Job drawing, mm, ordinate dimensions from the low corner. One solid piece. Round coordinates to 2 decimals unless told otherwise and drop trailing zeros. Write each loop counter-clockwise with the first axis right and the second up, starting at its lowest first coordinate (ties: lowest second). Pieces come first, ordered by that corner, then holes.
1) Saw through at D-D (z = 43.5). Write the cut outline in (x, y).
2) Saw through at C-C (z = 23). Write the cut outline in (x, y), plus the area to 3 significant figures.
3) Saw through at A-A (x = 1.1). State how many separate pieces and enclosed holes the cut face has, plus the area to 3 significant figures.
4) Saw through at B-B (y = 37). Write the cut outline in (x, z).
5) Flat gauge pins, fed straight in: pin 1 (1.5 mm diameter, centred on x = 2.5, y = 30.5, fed in from +Z); pin 2 (2 mm diameter, centred on y = 35, z = 7, fed in from -X). Where does each tip first touch, or does it go through?
6) Wall check: probe 1 along Y at (x, z) = (1.95, 23); probe 2 along Z at (x, y) = (0.9, 23.5); probe 3 along Y at (x, z) = (2.2, 10). Give the ranges that are in metal, low to high.
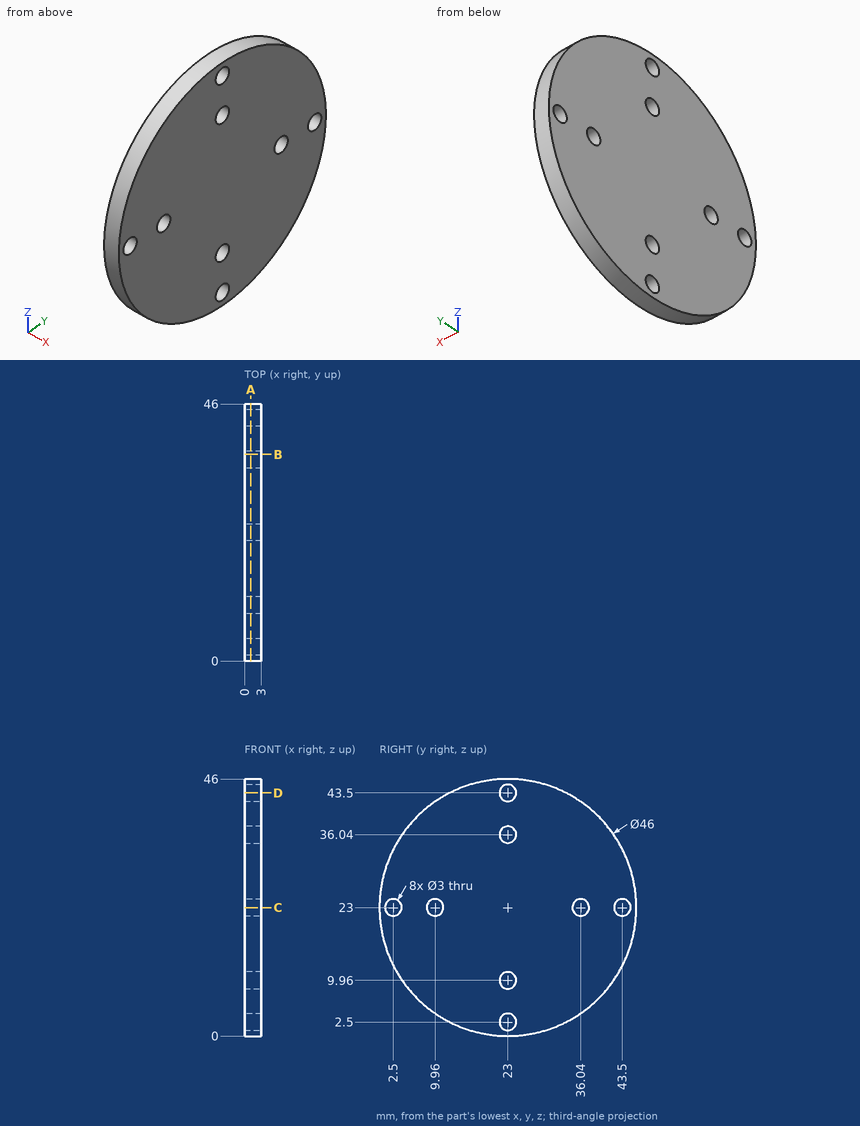
Evaluation:
1. outline: (0, 12.57) - (3, 12.57) - (3, 21.5) - (0, 21.5) - close; (0, 24.5) - (3, 24.5) - (3, 33.43) - (0, 33.43) - close
2. outline: (0, 0) - (3, 0) - (3, 1) - (0, 1) - close; (0, 4) - (3, 4) - (3, 8.46) - (0, 8.46) - close; (0, 11.46) - (3, 11.46) - (3, 34.54) - (0, 34.54) - close; (0, 37.54) - (3, 37.54) - (3, 42) - (0, 42) - close; (0, 45) - (3, 45) - (3, 46) - (0, 46) - close
2. area: 102 mm2
3. separate pieces: 1
3. enclosed holes: 8
3. area: 1,610 mm2
4. outline: (0, 4.75) - (3, 4.75) - (3, 21.85) - (0, 21.85) - close; (0, 24.15) - (3, 24.15) - (3, 41.25) - (0, 41.25) - close
5. pin 1: stops at z = 44.99
5. pin 2: stops at x = 0
6. probe 1: y = 0 to 1, 4 to 8.46, 11.46 to 34.54, 37.54 to 42, 45 to 46
6. probe 2: z = 0.01 to 1.09, 3.91 to 8.55, 11.37 to 34.63, 37.45 to 42.09, 44.91 to 45.99
6. probe 3: y = 4.03 to 21.5, 24.5 to 41.97
